Could you check a few things on this model? Use its own coordinates, in mm. Face numbers are marked on the shaded views. A direction names the side the tool comes from. Give positions to 0.01 mm unless a question says otherwise; leave off trailing zeros. Order: outer loops, then holes, each group sorted by start corner. A loop starts at its lowest first (then second) coordinate and runs counter-clockwise, first axis right, second up. Notation, with made-up numbers: (58.5, 21.25) -> (95.5, 21.25) arc R7 ccw to (95.5, 26.25) -> close; hole circle Ø1 at (6.5, 88). An arc over 180 degrees is marked (long way). One line per item, written item: value.
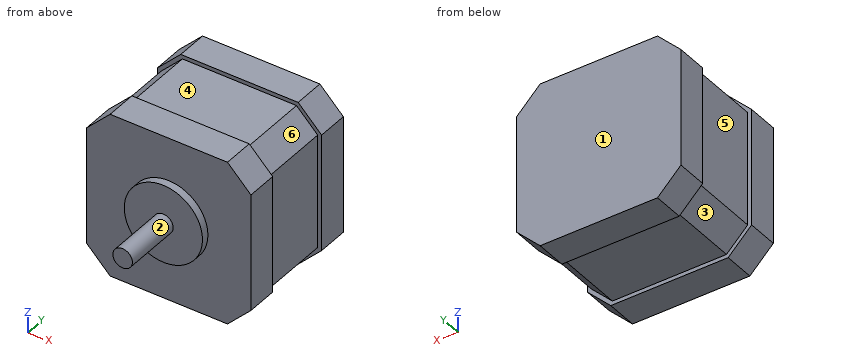
```python
from build123d import *

# Parameters (mm, degrees)
F0_W     = 42
F0_H     = 42
F1_DEPTH = 34
F2_SIZE  = 6
F5_DEPTH = 18
F6_R     = 10
F7_DEPTH = 2
F8_R     = 2.5
F9_DEPTH = 15


with BuildPart() as f1:
    # F0 (on Front) → F1 (new body)
    with BuildSketch(Plane.XZ):
        Rectangle(F0_W, F0_H)
    extrude(amount=-F1_DEPTH)

    # F2
    f2_edges = [f1.edges().sort_by_distance(p)[0] for p in [
        (21, 17, 21),
        (-21, 17, 21),
        (21, 17, -21),
        (-21, 17, -21),
    ]]
    chamfer(f2_edges, length=F2_SIZE)

    # F4 (on offset) → F5 (cut)
    with BuildSketch(Plane.XZ.offset(-8)):
        Polygon((15, 21), (-15, 21), (-21, 15), (-21, -15), (-15, -21), (15, -21), (21, -15), (21, 15), align=None)
        Polygon((-20, 14.585786), (-14.585786, 20), (14.585786, 20), (20, 14.585786), (20, -14.585786), (14.585786, -20), (-14.585786, -20), (-20, -14.585786), align=None, mode=Mode.SUBTRACT)
    extrude(amount=-F5_DEPTH, mode=Mode.SUBTRACT)

    # F6 (on Front) → F7 (join)
    with BuildSketch(Plane.XZ):
        Circle(F6_R)
    extrude(amount=F7_DEPTH)

    # F8 (on face) → F9 (join)
    with BuildSketch(Plane.XZ.offset(2)):
        Circle(F8_R)
    extrude(amount=F9_DEPTH)


solid = f1.part
```
1) We'd pull the mould along Y, two halves only. Please class the marked faces 1, 2 and 3: +Y half, -Y half, draft (parallel to the pull), parting line (faces both ways), or undercut.
Answer below:
face 1: +Y half
face 2: draft
face 3: undercut
2) Suppose I cut it at D-D, the plane z = 8. Write out the boundary of the cut face in (x, y), then the cut area to 3 significant figures.
Answer below:
outline: (-21, 0) -> (-6, 0) -> (-6, -2) -> (6, -2) -> (6, 0) -> (21, 0) -> (21, 8) -> (20, 8) -> (20, 26) -> (21, 26) -> (21, 34) -> (-21, 34) -> (-21, 26) -> (-20, 26) -> (-20, 8) -> (-21, 8) -> close
area: 1,420 mm2
3) Suppose I cut it at C-C, the plane x = 0. Write out the boundary of the cut face in (y, z), then the cut area to 3 significant figures.
Answer below:
outline: (-17, -2.5) -> (-2, -2.5) -> (-2, -10) -> (0, -10) -> (0, -21) -> (8, -21) -> (8, -20) -> (26, -20) -> (26, -21) -> (34, -21) -> (34, 21) -> (26, 21) -> (26, 20) -> (8, 20) -> (8, 21) -> (0, 21) -> (0, 10) -> (-2, 10) -> (-2, 2.5) -> (-17, 2.5) -> close
area: 1,510 mm2
4) Suppose I cut it at B-B, the plane y = 17. Write out the boundary of the cut face in (x, z), then the cut area to 3 significant figures.
Answer below:
outline: (-20, -14.59) -> (-14.59, -20) -> (14.59, -20) -> (20, -14.59) -> (20, 14.59) -> (14.59, 20) -> (-14.59, 20) -> (-20, 14.59) -> close
area: 1,540 mm2
5) Suppose I cut it at A-A, the plane z = 0. Write out the boundary of the cut face in (x, y), then the cut area to 3 significant figures.
Answer below:
outline: (-21, 0) -> (-10, 0) -> (-10, -2) -> (-2.5, -2) -> (-2.5, -17) -> (2.5, -17) -> (2.5, -2) -> (10, -2) -> (10, 0) -> (21, 0) -> (21, 8) -> (20, 8) -> (20, 26) -> (21, 26) -> (21, 34) -> (-21, 34) -> (-21, 26) -> (-20, 26) -> (-20, 8) -> (-21, 8) -> close
area: 1,510 mm2
6) If I drill on line 1 along Y through (x, z) = (9.5, -15.5); line 2 along X through (y, z) = (18.5, -6.5); line 3 along Y through (x, z) = (-3.5, 5.5), over which ranges is the centre line in solid material (lowest first)?
Answer below:
line 1: y = 0 to 34
line 2: x = -20 to 20
line 3: y = -2 to 34
7) For P1, Ø1, axis at x = 16, y = 27, coming from the +Z side; P2, Ø5.5, axis at x = 6, y = 16.5, coming from the +Z side; P3, Ø5.5, axis at x = -4.5, y = 16.5, coming from the -Z side, each with a flat end and sliding along its axis, tell me the tip position at first contact or that it passes through.
Answer below:
P1: stops at z = 20.5
P2: stops at z = 20
P3: stops at z = -20
8) For the marked faces 4, 5 and 6, which set-ups out of +Z, -Z, +X, -X, +Y, -Y let a thin tool reach every point of the face, with its end or its side?
Answer below:
face 4: +Z, +X, -X
face 5: +Z, -Z, -X
face 6: +Z, +X
